from build123d import *

# Parameters (mm, degrees)
SKETCH1_R                 = 60
BOSS_EXTRUDE1_DEPTH       = 20
BOSS_EXTRUDE1_DRAFT       = -40
SHELL1_T                  = -5
SKETCH3_W                 = 27
SKETCH3_H                 = 21
BOSS_EXTRUDE2_DEPTH       = 6
F_3_0MM_DOWEL_HOLE1_D     = 3
F_3_0MM_DOWEL_HOLE1_DEPTH = 4
F_3_0MM_DOWEL_HOLE1_TIP   = 0.901290929
F_3_0MM_DOWEL_HOLE2_D     = 3
F_3_0MM_DOWEL_HOLE2_DEPTH = 10
F_3_0MM_DOWEL_HOLE2_TIP   = 0.901290929
FILLET2_R                 = 2
F_3_0MM_DOWEL_HOLE3_D     = 3
F_3_0MM_DOWEL_HOLE3_DEPTH = 4
F_3_0MM_DOWEL_HOLE3_TIP   = 0.901290929
CUT_EXTRUDE1_DEPTH        = 10
FILLET3_R                 = 3


with BuildPart() as part:
    # Sketch1 → Boss-Extrude1 (with draft: the straight prism first)
    with BuildSketch(Plane(origin=(0, 0, 0), x_dir=(1, 0, 0), z_dir=(0, 1, 0))):
        Circle(SKETCH1_R)
    extrude(amount=-BOSS_EXTRUDE1_DEPTH)
    # Boss-Extrude1: the draft: its side faces are tilted about the plane it starts from
    boss_extrude1_sides = [part.faces().sort_by_distance(p)[0] for p in [
        (-60, -10, 0),
    ]]
    draft(boss_extrude1_sides, Plane(origin=(0, 0, 0), x_dir=(1, 0, 0), z_dir=(0, 1, 0)), BOSS_EXTRUDE1_DRAFT)

    # Shell1
    shell1_openings = [part.faces().sort_by_distance(p)[0] for p in [
        (0, 0, 0),
    ]]
    offset(amount=SHELL1_T, openings=shell1_openings, kind=Kind.INTERSECTION)

    # Sketch3 → Boss-Extrude2 (add)
    with BuildSketch(Plane(origin=(0, -15, 0), x_dir=(1, 0, 0), z_dir=(0, 1, 0))):
        Rectangle(SKETCH3_W, SKETCH3_H)
        with BuildLine():
            Line((-11, 8.5), (11, 8.5))
            ThreePointArc((11, 8.5), (11.353553391, 8.353553391), (11.5, 8))
            Line((11.5, 8), (11.5, -8))
            ThreePointArc((11.5, -8), (11.353553391, -8.353553391), (11, -8.5))
            Line((11, -8.5), (-11, -8.5))
            ThreePointArc((-11, -8.5), (-11.353553391, -8.353553391), (-11.5, -8))
            Line((-11.5, -8), (-11.5, 8))
            ThreePointArc((-11.5, 8), (-11.353553391, 8.353553391), (-11, 8.5))
        make_face(mode=Mode.SUBTRACT)
    extrude(amount=BOSS_EXTRUDE2_DEPTH)

    # Ø3.0mm Dowel Hole1
    with Locations(Plane(origin=(0, -15, 0), x_dir=(1, 0, 0), z_dir=(0, 1, 0))):
        with Locations((-29.999119987, 17.32), (29.999119987, 17.32), (0, -34.64)):
            Hole(F_3_0MM_DOWEL_HOLE1_D / 2, depth=F_3_0MM_DOWEL_HOLE1_DEPTH)
            with Locations((0, 0, -(F_3_0MM_DOWEL_HOLE1_DEPTH + F_3_0MM_DOWEL_HOLE1_TIP / 2))):  # 118° drill point
                Cone(0, F_3_0MM_DOWEL_HOLE1_D / 2, F_3_0MM_DOWEL_HOLE1_TIP, mode=Mode.SUBTRACT)

    # Ø3.0mm Dowel Hole2
    with Locations(Plane(origin=(0, -15, 0), x_dir=(1, 0, 0), z_dir=(0, 1, 0))):
        with Locations((4.5, 5.5), (4.5, -6.5)):
            Hole(F_3_0MM_DOWEL_HOLE2_D / 2, depth=F_3_0MM_DOWEL_HOLE2_DEPTH)
            with Locations((0, 0, -(F_3_0MM_DOWEL_HOLE2_DEPTH + F_3_0MM_DOWEL_HOLE2_TIP / 2))):  # 118° drill point
                Cone(0, F_3_0MM_DOWEL_HOLE2_D / 2, F_3_0MM_DOWEL_HOLE2_TIP, mode=Mode.SUBTRACT)

    # Fillet2
    fillet2_edges = [part.edges().sort_by_distance(p)[0] for p in [
        (-13.5, -15, 0),
        (0, -15, 10.5),
        (13.5, -15, 0),
        (0, -15, -10.5),
    ]]
    fillet(fillet2_edges, radius=FILLET2_R)

    # Ø3.0mm Dowel Hole3
    with Locations(Plane(origin=(0, -20, 0), x_dir=(-1, 0, 0), z_dir=(0, -1, 0))):
        with Locations((0, -19), (-16.454482672, 9.5), (16.454482672, 9.5)):
            Hole(F_3_0MM_DOWEL_HOLE3_D / 2, depth=F_3_0MM_DOWEL_HOLE3_DEPTH)
            with Locations((0, 0, -(F_3_0MM_DOWEL_HOLE3_DEPTH + F_3_0MM_DOWEL_HOLE3_TIP / 2))):  # 118° drill point
                Cone(0, F_3_0MM_DOWEL_HOLE3_D / 2, F_3_0MM_DOWEL_HOLE3_TIP, mode=Mode.SUBTRACT)

    # Sketch11 → Cut-Extrude1 (cut)
    with BuildSketch(Plane.XZ.offset(20)):
        Polygon((0.341916748, -5.046701194), (-2.228267182, -6.594006776), (-6.87018393, 1.116545014), (-4.3, 2.663850596), align=None)
    extrude(amount=-CUT_EXTRUDE1_DEPTH, mode=Mode.SUBTRACT)

    # Fillet3
    fillet3_edges = [part.edges().sort_by_distance(p)[0] for p in [
        (-40.886469086, -15, 0),
    ]]
    fillet(fillet3_edges, radius=FILLET3_R)


solid = part.part
Build history of the part. All positions in model axes, mm. A direction names the side the tool comes from. Give positions to 0.01 mm unless a question says otherwise; leave off trailing zeros. Order: outer loops, then holes, each group sorted by start corner. A loop starts at its lowest first (then second) coordinate and runs counter-clockwise, first axis right, second up. Notation, with made-up numbers: M -9,-23.75 L 1,-23.75 A17 cw 1,8.25 Z; hole C 76,16 d9. An arc over 180 degrees is marked long. Use one line per item in the form item = value.
1) Probe probe 1 along X at (y, z) = (-18.75, -9.5); probe 2 along Z at (x, y) = (9.5, -11.5); probe 3 along Y at (x, z) = (-20, 16). List the from-to ranges inside material, lowest first.
Calculated:
probe_1 = -43.24 to -17.95, -14.95 to 14.95, 17.95 to 43.24
probe_2 = -49.45 to -42.78, -10.5 to -8.5, 8.5 to 10.5, 42.78 to 49.45
probe_3 = -20 to -15
2) Saw through at A-A (y = -11.25). Give the cut face in (x, z).
Calculated:
outline = C 0,0 d101.12; M -13.5,-10.5 L 13.5,-10.5 L 13.5,10.5 L -13.5,10.5 Z; hole C 0,0 d88.07; hole M -11.5,-8 A0.5 ccw -11,-8.5 L 11,-8.5 A0.5 ccw 11.5,-8 L 11.5,8 A0.5 ccw 11,8.5 L -11,8.5 A0.5 ccw -11.5,8 Z
3) Tool access for faces 1 (the face through (-5.6, -17.54, 1.88)), 2 (the face through (15.26, -17.97, -8.59)), 3 (the face through (-11.5, -12, 0)): list every direction of +Z, -Z, +X, -X, +Y, -Y with a clear straight run to the whole face (end or side of a thin tool).
Calculated:
face_1 = +Y, -Y
face_2 = -Y
face_3 = +Y
4) Drop flat-ended pins along their axis: pin 1 (5 mm diameter, centred on x = 4.5, z = 6.5, fed in from +Y); pin 2 (1 mm diameter, centred on y = -12, z = 8, fed in from +X); pin 3 (3 mm diameter, centred on y = -12, z = 3.5, fed in from -X). Give the stop position or say it passes through.
Calculated:
pin_1 = -9
pin_2 = 49.72
pin_3 = -51.07
